```python
from build123d import *

# Parameters (mm, degrees)
F1_DEPTH  = 63.5
F2_DEPTH  = 25.4
F3_DEPTH  = 7.9375
F2_FACE_W = 50.8
F2_FACE_H = 19.05
F4_DEPTH  = 25.4
F6_R      = 6.35


with BuildPart() as f1:
    # F0 (on Front) → F1 (new body, symmetric)
    with BuildSketch(Plane.XZ):
        Polygon((-47.625, -9.525), (47.625, -9.525), (47.625, 9.525), (28.575, 9.525), (-47.625, 9.525), align=None)
    extrude(amount=F1_DEPTH, both=True)

    # F0 (on Front) → F2 (join, symmetric)
    with BuildSketch(Plane.XZ):
        with BuildLine():
            Line((28.575, 9.525), (47.625, 9.525))
            Line((47.625, 9.525), (47.625, 27.0002))
            ThreePointArc((47.625, 27.0002), (52.27468, 38.22552), (63.5, 42.8752))
            Line((63.5, 42.8752), (66.675, 42.8752))
            Line((66.675, 42.8752), (66.675, 61.9252))
            Line((66.675, 61.9252), (63.5, 61.9252))
            ThreePointArc((63.5, 61.9252), (38.804296, 51.695904), (28.575, 27.0002))
            Line((28.575, 27.0002), (28.575, 9.525))
        make_face()
    extrude(amount=F2_DEPTH, both=True)

    # F0 (on Front) → F3 (join, symmetric)
    with BuildSketch(Plane.XZ):
        with BuildLine():
            add(Edge.make_bspline(
                [(-47.625, 9.525), (-47.097944, 30.442789), (0, 62.250186), (63.5, 61.9252)],
                knots=[0, 0, 0, 0, 122.859866, 122.859866, 122.859866, 122.859866], degree=3))
            Line((-47.625, 9.525), (28.575, 9.525))
            Line((28.575, 9.525), (28.575, 27.0002))
            ThreePointArc((28.575, 27.0002), (38.804296, 51.695904), (63.5, 61.9252))
        make_face()
    extrude(amount=F3_DEPTH, both=True)

    # F2_face (on face) → F4 (join)
    with BuildSketch(Plane(origin=(66.675, 0, 52.4002), x_dir=(0, 1, 0), z_dir=(1, 0, 0))):
        Rectangle(F2_FACE_W, F2_FACE_H)
    extrude(amount=F4_DEPTH)

    # F0 (on Front) → F5 (revolve)
    with BuildSketch(Plane.XZ):
        Polygon((91.912158, 66.675), (91.912158, 61.9252), (91.912158, 42.8752), (91.912158, 38.1), (117.475, 38.1), (117.475, 66.675), align=None)
    revolve(axis=Axis((91.912158, 0, 52.3875), (0, 0, -1)))

    # F6
    f6_edges = [f1.edges().sort_by_distance(p)[0] for p in [
        (47.625, 63.5, 0),
        (-47.625, 63.5, 0),
        (-47.625, -63.5, 0),
        (47.625, -63.5, 0),
    ]]
    fillet(f6_edges, radius=F6_R)


solid = f1.part
```
Verification items for the finished model (mm, model axes). A direction names the side the tool comes from. Give positions to 0.01 mm unless a question says otherwise; leave off trailing zeros. Order: outer loops, then holes, each group sorted by start corner. A loop starts at its lowest first (then second) coordinate and runs counter-clockwise, first axis right, second up. Notation, with made-up numbers: (57.25, 10.25) -> (111.25, 10.25) arc R22 cw to (111.25, 29.25) -> close; hole circle Ø9 at (58.5, -35.75). An arc over 180 degrees is marked (long way). Use a Markdown table: item, result.
1) Section check A-A, the plane y = -14. Record the boundary of the cut face in (x, z) (3 decimals).
Results:
| item | result |
|---|---|
| outline | (-47.625, -9.525) -> (47.625, -9.525) -> (47.625, 27) arc R15.875 cw to (63.5, 42.875) -> (70.524, 42.875) -> (70.524, 38.1) -> (113.3, 38.1) -> (113.3, 66.675) -> (70.524, 66.675) -> (70.524, 61.925) -> (63.5, 61.925) arc R34.925 ccw to (28.575, 27) -> (28.575, 9.525) -> (-47.625, 9.525) -> close |
2) Material ranges on probe 1 along Z at (x, y) = (14, -29) (3 decimals); probe 2 along X at (y, z) = (-20, 22.5) (3 decimals); probe 3 along Y at (x, z) = (-22.5, 31.5), recorded low to high.
Results:
| item | result |
|---|---|
| probe 1 | -9.525 to 9.525 |
| probe 2 | 28.575 to 47.625 |
| probe 3 | -7.94 to 7.94 |
3) Depth check by flat-ended pin: pin 1 Ø12 at (x, z) = (4, 39) entering from -Y; pin 2 Ø3 at (y, z) = (-8, 16) entering from +X (3 decimals); pin 3 Ø2 at (x, y) = (8.5, 14.5) entering from +Z (3 decimals). Enter the tip coordinate at first touch or a pass-through.
Results:
| item | result |
|---|---|
| pin 1 | y = -7.94 |
| pin 2 | x = 47.625 |
| pin 3 | z = 9.525 |
4) Section check C-C, the plane x = 102. Record the boundary of the cut face in (y, z) (3 decimals).
Results:
| item | result |
|---|---|
| outline | (-23.488, 38.1) -> (23.488, 38.1) -> (23.488, 66.675) -> (-23.488, 66.675) -> close |
5) Section check B-B, the plane x = 80.5. Record the boundary of the cut face in (y, z) (3 decimals).
Results:
| item | result |
|---|---|
| outline | (-25.4, 42.875) -> (-22.874, 42.875) -> (-22.874, 38.1) -> (22.874, 38.1) -> (22.874, 42.875) -> (25.4, 42.875) -> (25.4, 61.925) -> (22.874, 61.925) -> (22.874, 66.675) -> (-22.874, 66.675) -> (-22.874, 61.925) -> (-25.4, 61.925) -> close |
6) Tool access check on faces 4 (the flat face through (66, 2, 61.925)), 5 (the flat face through (-4, -7.938, 30)), 6 (the flat face through (66, 2, 42.875)), 7 (the flat face through (52, 25.4, 41)). Record the directions out of +Z, -Z, +X, -X, +Y, -Y that give a thin tool (end or side, any length) a straight path to the whole face; none if there is none.
Results:
| item | result |
|---|---|
| face 4 | +Z, -X |
| face 5 | +Z, -X, -Y |
| face 6 | -Z |
| face 7 | +Z, -X, +Y |
7) Mould release check, pull along X, two halves, no side actions. Record for faces 1 (the flat face through (47.625, -1, 4)), 2 (the flat face through (-4, 7.938, 30)), 3 (the cylindrical face through (52.15, -0.36, 38.1)): pulls with the +X half, pulls with the -X half, needs draft (parallel to the pull), parting line crosses it, or undercut.
Results:
| item | result |
|---|---|
| face 1 | pulls with the +X half |
| face 2 | needs draft |
| face 3 | undercut |
